CAD build for the part. Positions are in the model's coordinates, mm. A direction names the side the tool comes from. Give positions to 0.01 mm unless a question says otherwise; leave off trailing zeros. Write each loop counter-clockwise with the first axis right and the second up, starting at its lowest first coordinate (ties: lowest second). Pieces come first, ordered by that corner, then holes. Notation, with made-up numbers: (81.25, -11.5) - (111.25, -11.5) arc R35 cw to (111.25, 26.5) - close; hole circle Ø8 at (36.25, 77.5). An arc over 180 degrees is marked (long way). Put each result on its own line as item: value. Start each with the question number.
1. Cut at C-C on y = 0. List the corners of the cut face in (x, z).
2. Wall check: line 1 (Y direction, x = -11, z = 0.8); line 2 (Z direction, x = -7.5, y = 2.5); line 3 (Z direction, x = 10.5, y = 6). Give the ranges that are in metal, low to high.
3. Mould opens along X. For faces 1 (the cylindrical face through (-12.2, -11.4, 0.5)), 2 (the cylindrical face through (9.76, -2.17, 2.48)), 3 (the flat face through (0, 0, 16)) say: +X half, -X half, draft (parallel to the pull), parting line (faces both ways), or undercut.
4. Drop flat-ended pins along their axis: pin 1 (8 mm diameter, centred on x = -3, y = 0, fed in from -Z); pin 2 (8 mm diameter, centred on y = -9.5, z = 13, fed in from +X); pin 3 (4 mm diameter, centred on x = -11, y = 10.5, fed in from +Z). Give the stop position or say it passes through.
5. Cut at A-A on x = 11. List the corners of the cut face in (y, z).
6. Cut at B-B on y = -10.5. List the corners of the cut face in (x, z), and give its area (3 significant figures).
7. Tool access for faces 4 (the cylindrical face through (7.81, -1.73, 14.99)), 5 (the flat face through (6, 4, 14)), 6 (the flat face through (-14.5, -0.2, 0.5)): list every direction of +Z, -Z, +X, -X, +Y, -Y with a clear straight run to the whole face (end or side of a thin tool).
8. Cut at D-D on x = 0. List the corners of the cut face in (y, z), and give its area (3 significant figures).
from build123d import *

# Parameters (mm, degrees)
SKETCH_1_W      = 29
SKETCH_1_H      = 26
SKETCH_1_R      = 1.5
EXTRUDE_1_DEPTH = 1


with BuildPart() as part:
    # 草图1 → 凸台-拉伸1 (new body)
    with BuildSketch(Plane.XY):
        Rectangle(SKETCH_1_W, SKETCH_1_H)
        with Locations((-11, 10.5)):
            Circle(SKETCH_1_R, mode=Mode.SUBTRACT)
        with Locations((11, 10.5)):
            Circle(SKETCH_1_R, mode=Mode.SUBTRACT)
        with Locations((11, -10.5)):
            Circle(SKETCH_1_R, mode=Mode.SUBTRACT)
        with Locations((-11, -10.5)):
            Circle(SKETCH_1_R, mode=Mode.SUBTRACT)
    extrude(amount=EXTRUDE_1_DEPTH)

    # 草图2 → 旋转2 (revolve)
    with BuildSketch(Plane(origin=(0, 0, 0), x_dir=(0, 0, -1), z_dir=(1, 0, 0))):
        Polygon((-1, 0), (-16, 0), (-16, 8), (-14, 8), (-14, 7), (-10, 7), (-10, 8), (-4, 8), (-4, 10), (-1, 10), align=None)
    revolve(axis=Axis((0, 0, 1), (0, 0, 1)))


solid = part.part
Report:
1. outline: (-14.5, 0) - (14.5, 0) - (14.5, 1) - (10, 1) - (10, 4) - (8, 4) - (8, 10) - (7, 10) - (7, 14) - (8, 14) - (8, 16) - (-8, 16) - (-8, 14) - (-7, 14) - (-7, 10) - (-8, 10) - (-8, 4) - (-10, 4) - (-10, 1) - (-14.5, 1) - close
2. line 1: y = -13 to -12, -9 to 9, 12 to 13
2. line 2: z = 0 to 10, 14 to 16
2. line 3: z = 0 to 1
3. face 1: undercut
3. face 2: parting line
3. face 3: draft
4. pin 1: stops at z = 0
4. pin 2: stops at x = 5.69
4. pin 3: stops at z = 1
5. outline: (-13, 0) - (-12, 0) - (-12, 1) - (-13, 1) - close; (-9, 0) - (9, 0) - (9, 1) - (-9, 1) - close; (12, 0) - (13, 0) - (13, 1) - (12, 1) - close
6. outline: (-14.5, 0) - (-12.5, 0) - (-12.5, 1) - (-14.5, 1) - close; (-9.5, 0) - (9.5, 0) - (9.5, 1) - (-9.5, 1) - close; (12.5, 0) - (14.5, 0) - (14.5, 1) - (12.5, 1) - close
6. area: 23.0 mm²
7. face 4: +Z
7. face 5: none
7. face 6: +Z, -Z, -X, +Y, -Y
8. outline: (-13, 0) - (13, 0) - (13, 1) - (10, 1) - (10, 4) - (8, 4) - (8, 10) - (7, 10) - (7, 14) - (8, 14) - (8, 16) - (-8, 16) - (-8, 14) - (-7, 14) - (-7, 10) - (-8, 10) - (-8, 4) - (-10, 4) - (-10, 1) - (-13, 1) - close
8. area: 270 mm²
